CAD build for the part. Positions are in the model's coordinates, mm. A direction names the side the tool comes from. Round coordinates to 2 decimals unless told otherwise and drop trailing zeros. Write each loop counter-clockwise with the first axis right and the second up, starting at its lowest first coordinate (ties: lowest second). Pieces come first, ordered by that corner, then holes. Notation, with made-up numbers: (62.5, -6) - (74.5, -6) arc R26 ccw to (74.5, 33) - close; hole circle Ø1 at (34.5, 49.25). An arc over 180 degrees is marked (long way). Put each result on its own line as item: value. Start each with the question number.
Item 1: 3-axis set-ups, long thin cutter, end or side, ignore diameter. For faces 1 (the flat face through (75, -48, -1)), 2 (the cylindrical face through (-85.09, -1.05, -84.615)), 3 (the cylindrical face through (-44.222, 43.982, 87.675)), 4 (the cylindrical face through (19.524, 49.86, -4.336)), 5 (the flat face through (75, 31, 55)): which of +Z, -Z, +X, -X, +Y, -Y reach the whole face in a straight line?
Item 2: Pin check, flat tips, straight feed: pin 1 Ø9.5 at (y, z) = (-49, 19) entering from +X; pin 2 Ø10 at (x, y) = (-78.5, 8) entering from +Z; pin 3 Ø10.5 at (y, z) = (46.5, 16) entering from -X. Stop position of each tip, or through.
Item 3: Drill centre lines: line 1 (Y direction, x = -72, z = -11.5); line 2 (Z direction, x = 0, y = 71); line 3 (Y direction, x = -29.5, z = -1). Where is each one in solid material? Low to high. Write a range as from..to.
Item 4: Cut at A-A (z = 0). Count the separate pieces of the cut face and the enclosed holes in it, and give its area (3 significant figures).
Item 5: Cut at D-D (x = 69.5). Give the cut face in (y, z), and give its area (3 significant figures).
Item 6: Mould opens along Z. For faces 6 (the flat face through (54, -31, 75)), 7 (the flat face through (-75, 29, 56)), 8 (the cylindrical face through (85.09, -1.05, 84.615)), 9 (the flat face through (-100, -51, -30.4)) say: released by +Z, released by -Z, zero draft, split by the parting line, or undercut.
Item 7: Cut at C-C (z = 36). Give the cut face in (x, y).
Autodesk Inventor part; units mm, degrees
ref_plane "YZ Plane" through (0, 0, 0) normal (1, 0, 0) x (0, 1, 0)
ref_plane "XZ Plane" through (0, 0, 0) normal (0, 1, 0) x (-1, 0, 0)
ref_plane "XY Plane" through (0, 0, 0) normal (0, 0, 1) x (1, 0, 0)
sketch "Sketch1" plane through (0, 0, 0) normal (0, 1, 0) x (-1, 0, 0)
  line L0 (-66.3325, -100) -> (66.3325, -100)
  line L1 (100, -66.3325) -> (100, 66.3325)
  line L2 (66.3325, 100) -> (-66.3325, 100)
  line L3 (-100, 66.3325) -> (-100, -66.3325)
  line L4 (-100, -100) -> (100, 100) construction
  line L5 (100, -100) -> (-100, 100) construction
  arc A0 (100, 66.3325) -> (66.3325, 100) centre (0, 0) ccw
  arc A1 (66.3325, -100) -> (100, -66.3325) centre (0, 0) ccw
  arc A2 (-66.3325, 100) -> (-100, 66.3325) centre (0, 0) ccw
  arc A3 (-100, -66.3325) -> (-66.3325, -100) centre (0, 0) ccw
  line L6 (60, 75) -> (-60, 75)
  line L7 (-75, 60) -> (-75, -60)
  line L8 (-60, -75) -> (60, -75)
  line L9 (75, -60) -> (75, 60)
  line L10 (75, 75) -> (-75, -75) construction
  line L11 (-75, 75) -> (75, -75) construction
  arc A4 (75, 60) -> (60, 75) centre (60, 60) ccw
  arc A5 (60, -75) -> (75, -60) centre (60, -60) ccw
  arc A6 (-75, -60) -> (-60, -75) centre (-60, -60) ccw
  arc A7 (-60, 75) -> (-75, 60) centre (-60, 60) ccw
  dimension "d0" = 200
  dimension "d1" = 200
  dimension "d3" = 150
  dimension "d4" = 150
  dimension "d5" = 15
extrude "Extrusion1" add sketch "Sketch1" along normal mid plane 150
sketch "Sketch2" plane through (0, 75, 0) normal (0, 1, 0) x (1, 0, 0)
  line L0 (66.3325, 100) -> (-66.3325, 100)
  line L1 (-100, 100) -> (-100, -66.3325)
  line L2 (-100, -100) -> (100, -100)
  line L3 (100, -66.3325) -> (100, 100)
  line L4 (100, 100) -> (-100, -100) construction
  line L5 (-100, 100) -> (100, -100) construction
  arc A0 (-100, -66.3325) -> (-66.3325, -100) centre (0, 0) ccw
  arc A1 (-66.3325, 100) -> (-100, 66.3325) centre (0, 0) ccw
  arc A2 (66.3325, -100) -> (100, -66.3325) centre (0, 0) ccw
  arc A3 (100, 66.3325) -> (66.3325, 100) centre (0, 0) ccw
  dimension "d8" = 200
  dimension "d9" = 200
extrude "Extrusion2" add sketch "Sketch2" against normal blind 35
hole "Hole1" at (0, 75, 0) direction (0, -1, 0) diameter 40 end through all
sketch "Sketch3" plane through (-66.3325, -75, 100) normal (0, 0, 1) x (1, 0, 0)
  line L0 (46.3325, 185) -> (86.3325, 185)
  line L1 (86.3325, 185) -> (86.3325, 135)
  line L2 (46.3325, 115) -> (46.3325, 185)
  line L3 (132.665, 150) -> (0, 150)
  line L4 (46.3325, 185) -> (86.3325, 115) construction
  line L5 (86.3325, 185) -> (46.3325, 115) construction
  line L6 (86.3325, 115) -> (86.3325, 150)
  line L7 (46.3325, 165) -> (86.3325, 165)
  line L8 (86.3325, 165) -> (86.3325, 135)
  line L9 (46.3325, 135) -> (46.3325, 165)
  line L10 (46.3325, 165) -> (86.3325, 135) construction
  line L11 (86.3325, 165) -> (46.3325, 135) construction
  line L12 (86.3325, 135) -> (66.3325, 78.4315)
  line L13 (86.3325, 115) -> (79.2614, 115)
  line L14 (66.3325, 115) -> (46.3325, 115)
  line L15 (86.3325, 135) -> (74.9039, 135)
  line L16 (66.3325, 135) -> (46.3325, 135)
  line L17 (66.3325, 75) -> (66.3325, 115)
  circle A0 centre (66.3325, 78.4315) radius 60
  point P0 (66.3325, 150)
  dimension "d21" = 40
  dimension "d22" = 70
  dimension "d23" = 30
  dimension "d24" = 60
extrude "Extrusion3" cut sketch "Sketch3" against normal blind 25 contours A0 L12 L17 L14 L2 | L2 L14 L17 L12 L13 L6 A0 | L6 L13 L12
mirror "Mirror1" about plane through (0, 0, 0) normal (0, 0, 1) of "Extrusion3"
sketch "Sketch4" plane through (-100, -75, -66.3325) normal (-1, 0, 0) x (0, 0, 1)
  line L0 (86.3325, 115) -> (86.3325, 150)
  line L1 (46.3325, 185) -> (86.3325, 185)
  line L2 (86.3325, 185) -> (86.3325, 132.5)
  line L3 (46.3325, 115) -> (46.3325, 185)
  line L4 (46.3325, 150) -> (86.3325, 150)
  line L5 (46.3325, 185) -> (86.3325, 115) construction
  line L6 (86.3325, 185) -> (46.3325, 115) construction
  line L7 (46.3325, 167.5) -> (86.3325, 167.5)
  line L8 (86.3325, 167.5) -> (86.3325, 132.5)
  line L9 (46.3325, 132.5) -> (46.3325, 167.5)
  line L10 (46.3325, 167.5) -> (86.3325, 132.5) construction
  line L11 (86.3325, 167.5) -> (46.3325, 132.5) construction
  line L12 (66.3325, 75) -> (66.3325, 115)
  line L13 (86.3325, 132.5) -> (66.3325, 75.9315)
  line L14 (86.3325, 132.5) -> (76.3325, 132.5)
  line L15 (56.3325, 132.5) -> (46.3325, 132.5)
  line L16 (66.3325, 115) -> (46.3325, 115)
  circle A0 centre (66.3325, 75.9315) radius 60
  point P0 (66.3325, 150)
  dimension "d27" = 60
extrude "Extrusion4" cut sketch "Sketch4" against normal blind 25 contours A0 L3 L16 L12 L13 | L13 L12 L16 L3 A0
mirror "Mirror2" about plane through (0, 0, 0) normal (1, 0, 0) of "Extrusion4"
sketch "Sketch5" plane through (0, 0, 0) normal (1, 0, 0) x (0, 1, 0)
  point P0 (0, 0)
sketch "Sketch6" plane through (0, -75, 0) normal (0, -1, 0) x (1, 0, 0)
  line L0 (-60, -75) -> (60, -75)
  line L1 (75, -60) -> (75, 60)
  line L2 (60, 75) -> (-60, 75)
  line L3 (-75, 60) -> (-75, -60)
  line L4 (-75, -75) -> (75, 75) construction
  line L5 (75, -75) -> (-75, 75) construction
  arc A0 (75, 60) -> (60, 75) centre (60, 60) ccw
  arc A1 (60, -75) -> (75, -60) centre (60, -60) ccw
  arc A2 (-75, -60) -> (-60, -75) centre (-60, -60) ccw
  arc A3 (-60, 75) -> (-75, 60) centre (-60, 60) ccw
  point P0 (0, 0)
  dimension "d21" = 40
  dimension "d30" = 150
  dimension "d31" = 150
  dimension "d32" = 15
extrude "Extrusion5" add sketch "Sketch6" against normal blind 35
hole "Hole2" at (0, -75, 0) direction (0, 1, 0) diameter 40 end through all
sketch "Sketch7" plane through (0, 0, 0) normal (0, 0, 1) x (1, 0, 0)
  line L0 (47.5683, 40) -> (-47.5683, 40)
  line L1 (66.3325, 75) -> (-66.3325, 75)
  point P0 (0, 0)
  point P1 (47.5683, 75)
sketch "Sketch8" plane through (0, 75, 0) normal (0, 1, 0) x (1, 0, 0)
  circle A0 centre (0, 0) radius 48.6322
extrude "Extrusion6" cut sketch "Sketch8" against normal blind 15
mirror "Mirror3" about plane through (0, 0, 0) normal (0, 1, 0) of "Extrusion6"
sketch "Sketch9" plane through (0, 0, 0) normal (0, 1, 0) x (-1, 0, 0)
  circle A0 centre (0, 0) radius 20
properties part number "hub"
Output values:
1. face 1: +X
1. face 2: -Z, -X, +Y, -Y
1. face 3: +Z
1. face 4: +Y, -Y
1. face 5: none
2. pin 1: x = 75
2. pin 2: z = 94.86
2. pin 3: x = -75
3. line 1: -75..-40, 40..75
3. line 2: -100..-48.63, 48.63..100
3. line 3: -60..-40, 40..60
4. separate pieces: 4
4. enclosed holes: 0
4. area: 7,480 mm2
5. outline: (-75, -97.83) - (75, -97.83) - (75, 97.83) - (-75, 97.83) - close; hole (-40, -71.61) - (40, -71.61) - (40, 71.61) - (-40, 71.61) - close
5. area: 17,900 mm2
6. face 6: undercut
6. face 7: undercut
6. face 8: released by +Z
6. face 9: zero draft
7. outline: (-100, -75) - (-32.7, -75) - (-32.7, -60) - (32.7, -60) - (32.7, -75) - (100, -75) - (100, -47.07) - (75, -47.07) - (75, -40) - (-75, -40) - (-75, -47.07) - (-100, -47.07) - close; (-100, 48.93) - (-75, 48.93) - (-75, 40) - (75, 40) - (75, 48.93) - (100, 48.93) - (100, 75) - (32.7, 75) - (32.7, 60) - (-32.7, 60) - (-32.7, 75) - (-100, 75) - close
